```python
from build123d import *

# Parameters (mm, degrees)
SKETCH_1_R          = 2.5
EXTRUDE_1_DEPTH     = 12
SKETCH_2_R          = 2
CUT_EXTRUDE_1_DEPTH = 5
SKETCH_3_R          = 1.5
EXTRUDE_2_DEPTH     = 4
FILLET_1_R          = 1.5


with BuildPart() as part:
    # 스케치1 → 보스-돌출1 (new body)
    with BuildSketch(Plane.XY):
        Polygon((6.588838908, 28.19675948), (4.588838908, -3.787132496), (-2.435084758, -9.224887606), (-6.651746097, -35.634279915), (-11.1649155, -35.634279915), (-9.242889687, -15.767948861), (-14.161167405, -15.767948861), (-14.558519827, -5.05323729), (-7, 0.71086224), (-2.849537727, 4.46912262), (-2.849537727, 10.047291676), (1.024768486, 10.047291676), (2.588838908, 27.569044976), align=None)
        Circle(SKETCH_1_R, mode=Mode.SUBTRACT)
    extrude(amount=EXTRUDE_1_DEPTH)

    # 스케치2 → 컷-돌출1 (cut)
    with BuildSketch(Plane(origin=(-0.938271737, 0.14980936, 0), x_dir=(0, 0, -1), z_dir=(0.9874921543617721, -0.1576681485714416, 0))):
        with Locations(Location((-6, -11.993439441, 0), (0, 0, 90))):
            Circle(SKETCH_2_R)
    extrude(amount=-CUT_EXTRUDE_1_DEPTH, mode=Mode.SUBTRACT)

    # 스케치3 → 보스-돌출2 (add)
    with BuildSketch(Plane(origin=(-5.875732509, 0.938150103, 0), x_dir=(0, 0, -1), z_dir=(0.9874921543617721, -0.1576681485714416, 0))):
        with Locations(Location((-6, -11.993439441, 0), (0, 0, 90))):
            Circle(SKETCH_3_R)
    extrude(amount=EXTRUDE_2_DEPTH)

    # 필렛1
    fillet_1_edges = [part.edges().sort_by_distance(p)[0] for p in [
        (-4.053249506, -13.017188075, 6),
    ]]
    fillet(fillet_1_edges, radius=FILLET_1_R)


solid = part.part
```
Build history of the part. All positions in model axes, mm. A direction names the side the tool comes from. Give positions to 0.01 mm unless a question says otherwise; leave off trailing zeros. Order: outer loops, then holes, each group sorted by start corner. A loop starts at its lowest first (then second) coordinate and runs counter-clockwise, first axis right, second up. Notation, with made-up numbers: M 48,46 L 97,46 A33 ccw 97,74 Z; hole C -12,70 d4. An arc over 180 degrees is marked long. Return JSON: item names as keys, results as strings.
Q1. Two-plate mould, pull along Y, no slides. Class faces 1 (the face through (-4, -4, 12)), 2 (the face through (-10.217, -25.84, 5.916)), 3 (the face through (-4.514, -22.245, 5.916)), 4 (the face through (4.56, 27.88, 5.92)): pulls with the +Y half, pulls with the -Y half, needs draft (parallel to the pull), parting line crosses it, or undercut.
Answer list:
{"face 1": "needs draft", "face 2": "undercut", "face 3": "pulls with the -Y half", "face 4": "pulls with the +Y half"}
Q2. Band-saw the part on A-A (z = 3.25). Give the cut face in (x, y).
Answer list:
{"outline": "M -14.56,-5.05 L -14.16,-15.77 L -9.24,-15.77 L -11.16,-35.63 L -6.65,-35.63 L -2.44,-9.22 L 4.59,-3.79 L 6.59,28.2 L 2.59,27.57 L 1.02,10.05 L -2.85,10.05 L -2.85,4.47 L -7,0.71 Z; hole C 0,0 d5"}
Q3. Band-saw the part on C-C (y = 0). Give the cut face in (x, z), then the cut area to 3 significant figures.
Answer list:
{"outline": "M -7.93,0 L -2.5,0 L -2.5,12 L -7.93,12 Z; M 2.5,0 L 4.83,0 L 4.83,12 L 2.5,12 Z", "area": "93.1 mm^2"}
Q4. Band-saw the part on B-B (x = 0). Give the cut face in (y, z).
Answer list:
{"outline": "M -7.34,0 L -2.5,0 L -2.5,12 L -7.34,12 Z; M 2.5,0 L 10.05,0 L 10.05,12 L 2.5,12 Z"}
Q5. Wall check: probe 1 along Z at (x, y) = (-4.5, -10.5); probe 2 along Y at (x, z) = (0, 6.75); probe 3 along Y at (x, z) = (-1.75, 1.5). Give the ranges that are in metal, low to high. Write a range as from..to.
Answer list:
{"probe 1": "z = 0..4.22, 5.01..6.99, 7.78..12", "probe 2": "y = -7.34..-2.5, 2.5..10.05", "probe 3": "y = -8.69..-1.79, 1.79..10.05"}
Q6. 3-axis set-ups, long thin cutter, end or side, ignore diameter. For faces 5 (the face through (-9, -35.634, 6)), 6 (the face through (-2.85, 7, 6)), 7 (the face through (-12, -15.768, 6)): which of +Z, -Z, +X, -X, +Y, -Y reach the whole face in a straight line?
Answer list:
{"face 5": "+Z, -Z, +X, -X, -Y", "face 6": "+Z, -Z, -X, +Y", "face 7": "+Z, -Z, -X"}
Q7. Flat gauge pins, fed straight in: pin 1 (1 mm diameter, centred on x = -11, y = -0.5, fed in from -Z); pin 2 (1.7 mm diameter, centred on y = 6.5, z = 9, fed in from -X); pin 3 (4 mm diameter, centred on x = 1.5, z = 7, fed in from +Y); pin 4 (1 mm diameter, centred on x = 0, z = 8.5, fed in from -Y). Where does each tip first touch, or does it go through?
Answer list:
{"pin 1": "passes through", "pin 2": "stops at x = -2.85", "pin 3": "stops at y = 27.71", "pin 4": "stops at y = -7.73"}
Q8. Band-saw the part on D-D (y = -20.5). Give the cut face in (x, z).
Answer list:
{"outline": "M -9.7,0 L -4.24,0 L -4.24,12 L -9.7,12 Z"}
